Geometry: final body of the model. Coordinates: model frame, mm. A direction names the side the tool comes from. Give positions to 0.01 mm unless a question says otherwise; leave off trailing zeros. Write each loop counter-clockwise with the first axis right and the second up, starting at its lowest first coordinate (ties: lowest second). Pieces come first, ordered by that corner, then holes. Notation, with made-up numbers: M -7.5,60 L 1.5,60 A29 cw 1.5,84 Z; hole C 12,-36 d8. An arc over 180 degrees is marked long. Answer as a JSON object with one key per item and string values.
from build123d import *

# Parameters (mm, degrees)
SKETCH1_R           = 4.5
SKETCH1_R_2         = 3.25
BOSS_EXTRUDE1_DEPTH = 20
SKETCH2_W           = 20
SKETCH2_H           = 10
BOSS_EXTRUDE2_DEPTH = 1.5
FILLET1_R           = 2
SKETCH2_4_W         = 20
SKETCH2_4_H         = 10
SKETCH2_4_R         = 2
BOSS_EXTRUDE3_DEPTH = 3
SKETCH4_R           = 45
CUT_EXTRUDE1_DEPTH  = 10


with BuildPart() as part:
    # Sketch1 → Boss-Extrude1 (new body)
    with BuildSketch(Plane(origin=(0, 0, 0), x_dir=(1, 0, 0), z_dir=(0, 1, 0))):
        with Locations(Location((0, 0, 0), (0, 0, 270))):
            Circle(SKETCH1_R)
        with Locations(Location((0, 0, 0), (0, 0, 270))):
            Circle(SKETCH1_R_2, mode=Mode.SUBTRACT)
    extrude(amount=BOSS_EXTRUDE1_DEPTH)

    # Sketch2 → Boss-Extrude2 (add, symmetric)
    with BuildSketch(Plane.XY.offset(-4.5)):
        with Locations((0, 15)):
            Rectangle(SKETCH2_W, SKETCH2_H)
    extrude(amount=BOSS_EXTRUDE2_DEPTH, both=True)

    # Fillet1
    fillet1_edges = [part.edges().sort_by_distance(p)[0] for p in [
        (-10, 10, -4.5),
        (10, 10, -4.5),
        (10, 20, -4.5),
        (-10, 20, -4.5),
    ]]
    fillet(fillet1_edges, radius=FILLET1_R)

    # Sketch2_4 → Boss-Extrude3 (add)
    with BuildSketch(Plane.XY.offset(-4.5)):
        with Locations((0, 15)):
            Rectangle(SKETCH2_4_W, SKETCH2_4_H)
        with Locations((-7.25, 15)):
            Circle(SKETCH2_4_R, mode=Mode.SUBTRACT)
        with Locations((7.25, 15)):
            Circle(SKETCH2_4_R, mode=Mode.SUBTRACT)
    extrude(amount=-BOSS_EXTRUDE3_DEPTH)

    # Sketch4 → Cut-Extrude1 (cut)
    with BuildSketch(Plane(origin=(0, 20, 0), x_dir=(1, 0, 0), z_dir=(0, 1, 0))):
        with Locations((0, 50.37974859)):
            Circle(SKETCH4_R)
    extrude(amount=-CUT_EXTRUDE1_DEPTH, mode=Mode.SUBTRACT)


solid = part.part
1) Cut plane B-B on x = 0. Return loops of the section in (y, z), and give its area (3 significant figures).
Geometry check:
{"outline": "M 0,-4.5 L 10,-4.5 L 10,-5.38 L 20,-5.38 L 20,-3 L 10,-3 L 10,-3.25 L 0,-3.25 Z; M 0,3.25 L 20,3.25 L 20,4.5 L 0,4.5 Z", "area": "61.3 mm2"}
2) Contact query for flat-ended pins moving along their axis: P1, Ø0.9, axis at x = 8, y = 14, coming from the -Z side; P2, Ø0.6, axis at x = 9.5, y = 19.5, coming from the +Z side; P3, Ø5, axis at x = 0, z = 0, coming from the -Y side; P4, Ø1.5, axis at x = 7, z = -4.5, coming from the -Y side. Output: stop coordinate, or through.
Geometry check:
{"P1": "stops at z = -6", "P2": "stops at z = -3", "P3": "passes through", "P4": "stops at y = 10"}
3) Cut plane C-C on y = 14.75. Return loops of the section in (x, z), and give its area (3 significant figures).
Geometry check:
{"outline": "M -10,-6.5 A45 cw -9.23,-6.34 L -9.23,-6 L -7.45,-6 A45 cw 7.45,-6 L 9.23,-6 L 9.23,-6.34 A45 cw 10,-6.5 L 10,-3 L 3.35,-3 A4.5 ccw long -3.35,-3 L -10,-3 Z; hole M -1.25,-3 L 1.25,-3 A3.25 ccw long Z", "area": "78.4 mm2"}
4) Line query: line 1 (Z direction, x = 0, y = 11); line 2 (Z direction, x = 0, y = 7). Output: solid intervals per line, ascending. Write a range as from..to.
Geometry check:
{"line 1": "z = -5.38..-3, 3.25..4.5", "line 2": "z = -4.5..-3.25, 3.25..4.5"}
5) Pull-direction query (Z, two-part tool) for faces 4 (the flat face through (0, 15, -3)), 5 (the flat face through (9.5, 19.6, -4.5)), 6 (the flat face through (-0.8, 20, -3.4)); classes: pulls with the +Z half, pulls with the -Z half, needs draft (parallel to the pull), parting line crosses it, or undercut.
Geometry check:
{"face 4": "undercut", "face 5": "pulls with the +Z half", "face 6": "needs draft"}
6) Set-up query: faces 1 (the flat face through (0, 10, -5)), 2 (the cylindrical face through (-9.43, 10.6, -3.74)), 3 (the cylindrical face through (9.25, 14.96, -6.17)). Return all of +Z, -Z, +X, -X, +Y, -Y with unobstructed straight access to the full face (end or side cutting, diameter ignored); none if empty.
Geometry check:
{"face 1": "-Z, -Y", "face 2": "+Z, -X, -Y", "face 3": "-Z"}
7) Cut plane A-A on z = 0. Return loops of the section in (x, y).
Geometry check:
{"outline": "M -4.5,0 L -3.25,0 L -3.25,20 L -4.5,20 Z; M 3.25,0 L 4.5,0 L 4.5,20 L 3.25,20 Z"}
8) Cut plane D-D on z = -2. Return loops of the section in (x, y).
Geometry check:
{"outline": "M -4.03,0 L -2.56,0 L -2.56,20 L -4.03,20 Z; M 2.56,0 L 4.03,0 L 4.03,20 L 2.56,20 Z"}
